Verification items for the finished model (mm, model axes). Face numbers are marked on the shaded views. A direction names the side the tool comes from. Coordinates: 2 decimals unless noted, no trailing zeros. Write each loop counter-clockwise with the first axis right and the second up, starting at its lowest first coordinate (ties: lowest second). Pieces come first, ordered by that corner, then holes. Notation, with made-up numbers: (-22.75, 25) -> (10.25, 25) arc R21 ccw to (10.25, 54) -> close; hole circle Ø7 at (43.5, -18). An arc over 180 degrees is marked (long way). Write item = value, one per line. Start each with the question number.
(1) Gauge pin test, flat ends, axial feed: pin 1 Ø2 at (x, z) = (13.5, 20) entering from -Y; pin 2 Ø5 at (y, z) = (4, 11.5) entering from +X; pin 3 Ø3 at (x, z) = (-13.5, 13.5) entering from +Y; pin 4 Ø12.5 at (x, z) = (-28, 10.5) entering from +Y. Record the tip position at first contact, or that the pin passes through.
(2) Material ranges on probe 1 along Y at (x, z) = (1.8, 9); probe 2 along Y at (x, z) = (-35, 18); probe 3 along Z at (x, y) = (17.5, 1), recorded low to high. Write a range as [from, to].
(3) Mould release check, pull along Z, two halves, no side actions. Record for the marked faces 4, 5, 6 and 7: released by +Z, released by -Z, zero draft, split by the parting line, or undercut.
(4) Section check C-C (x = 7). Record the cut outline in (y, z), plus the area to 3 significant figures.
(5) Section check A-A (x = -23). Record the cut outline in (y, z).
(6) Section check D-D (y = -11.5). Record the cut outline in (x, z).
(7) Section check B-B (z = 12.5). Record the cut outline in (x, y), plus the area to 3 significant figures.
(8) Set-up check for the marked faces 1, 2 and 3: record each of +Z, -Z, +X, -X, +Y, -Y from which the full face is reachable in a straight line by a thin tool's end or side.
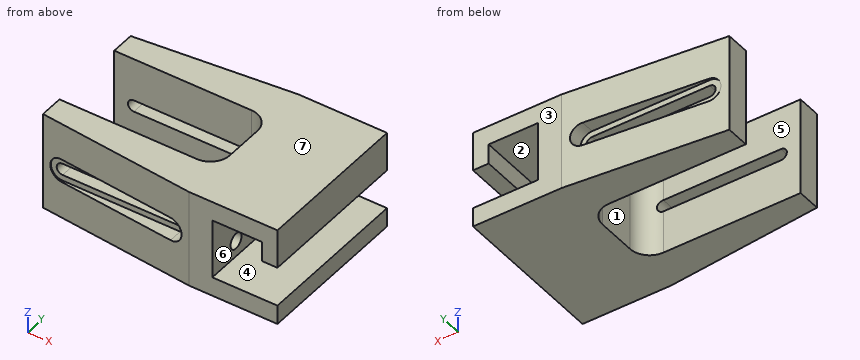
Autodesk Inventor part; units mm, degrees
ref_plane "Work Plane1" through (-40, -10, 25) normal (0, 1, 0) x (1, 0, 0)
ref_plane "YZ Plane" through (0, 0, 0) normal (1, 0, 0) x (0, 1, 0)
ref_plane "XZ Plane" through (0, 0, 0) normal (0, 1, 0) x (-1, 0, 0)
sketch "Sketch1" plane through (0, 0, 0) normal (0, 0, 1) x (1, 0, 0)
  line L0 (-40, 0) -> (0, 0)
  line L1 (0, 0) -> (0, -20)
  line L2 (0, -20) -> (-40, -20)
  line L3 (-40, -20) -> (-40, -26)
  line L4 (-40, -26) -> (0, -30)
  line L5 (0, -30) -> (6, -30)
  line L6 (6, -30) -> (6, 10)
  line L7 (6, 10) -> (0, 10)
  line L8 (0, 10) -> (-40, 6)
  line L9 (-40, 6) -> (-40, 0)
  dimension "d0" = 6
  dimension "d1" = 40
  dimension "d2" = 20
  dimension "d3" = 40
extrude "Extrusion1" add sketch "Sketch1" along normal blind 25
sketch "Sketch2" plane through (6, -30, 0) normal (1, 0, 0) x (0, 0, -1)
  line L0 (0, 40) -> (-25, 40)
  line L1 (0, 0) -> (-25, 0)
  line L2 (-25, 40) -> (-20, 40)
  line L3 (-20, 40) -> (-20, 0)
  line L4 (-20, 0) -> (-25, 0)
  line L5 (-25, 0) -> (-25, 40)
  line L6 (0, 0) -> (-5, 0)
  line L7 (-5, 0) -> (-5, 40)
  line L8 (-5, 40) -> (0, 40)
  line L9 (0, 40) -> (0, 0)
  circle A0 centre (-9, 8.6346) radius 1.7
  line L10 (-2.5, 11.8846) -> (-2.5, 5.3846)
  point P0 (0, 30)
  point P1 (-25, 0)
  point P2 (-5, 0)
  dimension "d6" = 5
  dimension "d7" = 5
  dimension "d30" = 4
  dimension "d31" = 8.6346
extrude "Extrusion2" add sketch "Sketch2" along normal blind 16.6 contours L9 L1 L7 L0 | L3 L1 L5 L0
hole "Hole2" at (6, -21.3654, 9) direction (-1, 0, 0) diameter 4 depth 6
sketch "Sketch3" plane through (0, 0, 0) normal (0, 0, -1) x (-1, 0, 0)
  line L0 (0, 0) -> (0, -20)
  arc A0 (0, -15) -> (5, -20) centre (5, -15) ccw
  arc A1 (5, 0) -> (0, -5) centre (5, -5) ccw
  line L1 (0, -20) -> (40, -20)
  line L2 (40, 0) -> (0, 0)
  dimension "d27" = 5
extrude "Extrusion3" add sketch "Sketch3" against normal up to surface (25 mm away)
sketch "Sketch4" plane through (0, 10, 25) normal (0, 1, 0) x (1, 0, 0)
  line L0 (-5, 12.5) -> (-35, 12.5) construction
  line L1 (-5, 9.5) -> (-35, 9.5)
  line L2 (-35, 15.5) -> (-5, 15.5)
  arc A0 (-5, 9.5) -> (-5, 15.5) centre (-5, 12.5) ccw
  arc A1 (-35, 15.5) -> (-35, 9.5) centre (-35, 12.5) ccw
  line L3 (-40, 25) -> (-40, 0)
  line L4 (0, 25) -> (0, 0)
  point P0 (-20, 12.5)
  point P1 (0, 12.5)
  dimension "d32" = 3
  dimension "d33" = 5
  dimension "d34" = 5
extrude "Extrusion4" cut sketch "Sketch4" against normal blind 4
sketch "Sketch5" plane through (0, 6, 25) normal (0, 1, 0) x (1, 0, 0)
  line L0 (-5, 12.5) -> (-35, 12.5) construction
  line L1 (-5, 14) -> (-35, 14)
  line L2 (-35, 11) -> (-5, 11)
  arc A0 (-5, 11) -> (-5, 14) centre (-5, 12.5) ccw
  arc A1 (-35, 14) -> (-35, 11) centre (-35, 12.5) ccw
  line L3 (-5, 9.5) -> (-35, 9.5)
  arc A2 (-5, 9.5) -> (-5, 15.5) centre (-5, 12.5) ccw
  line L4 (-35, 15.5) -> (-5, 15.5)
  arc A3 (-35, 15.5) -> (-35, 9.5) centre (-35, 12.5) ccw
  point P0 (0, 25)
  point P1 (-20, 12.5)
  dimension "d37" = 1.5
extrude "Extrusion5" cut sketch "Sketch5" against normal blind 10.75 contours A0 L2 A1 L1
ref_plane "Work Plane1" through (-40, -10, 25) normal (0, 1, 0) x (1, 0, 0)
mirror "Mirror1" about plane through (-40, -10, 25) normal (0, 1, 0) of "Extrusion4", "Extrusion5", "Hole2"
sketch "Sketch6" plane through (6, -30, 20) normal (0, 0, -1) x (-1, 0, 0)
  line L0 (0, 40) -> (0, 0)
  line L1 (0, 40) -> (-16.6, 40)
  line L2 (-16.6, 0) -> (-16.6, 40)
  line L3 (0, 0) -> (-16.6, 0)
  line L4 (-16.6, 40) -> (-16.6, 0)
  line L5 (0, 0) -> (-16.6, 0)
  line L6 (-16.6, 40) -> (-12.6, 40)
  line L7 (-12.6, 40) -> (-12.6, 0)
  line L8 (-12.6, 0) -> (-16.6, 0)
  line L9 (-16.6, 0) -> (-16.6, 40)
  point P0 (6, 30)
  dimension "d40" = 4
extrude "Extrusion6" add sketch "Sketch6" along normal blind 5 contours L7 L3 L2 L1
thicken "Thicken1" operation add thickness 0.1 both sides no extend neighbours yes toward (0, 0, 1) faces at (14.4, -3.3333, 20) (11.5333, -3.3333, 5)
properties part number "Z Belt 2"
Response:
q1.pin_1 = -30
q1.pin_2 = 6
q1.pin_3 = 6
q1.pin_4 = 7.82
q2.probe_1 = [-30, -23.37], [-19.37, -0.63], [3.37, 10]
q2.probe_2 = [-26.5, -20], [0, 6.5]
q2.probe_3 = [0, 4.9], [20.1, 25]
q3.face_4 = undercut
q3.face_5 = zero draft
q3.face_6 = undercut
q3.face_7 = released by +Z
q4.outline = (-30, 0) -> (10, 0) -> (10, 4.9) -> (-30, 4.9) -> close; (-30, 20.1) -> (10, 20.1) -> (10, 25) -> (-30, 25) -> close
q4.area = 392 mm2
q5.outline = (-27.7, 0) -> (-20, 0) -> (-20, 11) -> (-26, 11) -> (-26, 9.5) -> (-27.7, 9.5) -> close; (-27.7, 15.5) -> (-26, 15.5) -> (-26, 14) -> (-20, 14) -> (-20, 25) -> (-27.7, 25) -> close; (0, 0) -> (7.7, 0) -> (7.7, 9.5) -> (6, 9.5) -> (6, 11) -> (0, 11) -> close; (0, 14) -> (6, 14) -> (6, 15.5) -> (7.7, 15.5) -> (7.7, 25) -> (0, 25) -> close
q6.outline = (0, 0) -> (22.6, 0) -> (22.6, 4.9) -> (6, 4.9) -> (6, 20.1) -> (18.6, 20.1) -> (18.6, 15) -> (22.6, 15) -> (22.6, 25) -> (0, 25) -> close
q7.outline = (-40, -26) -> (-38, -26.2) -> (-38, -26) -> (-36.5, -26) -> (-36.5, -20) -> (-40, -20) -> close; (-40, 0) -> (-36.5, 0) -> (-36.5, 6) -> (-38, 6) -> (-38, 6.2) -> (-40, 6) -> close; (-3.5, -26) -> (-2, -26) -> (-2, -29.8) -> (0, -30) -> (6, -30) -> (6, 10) -> (0, 10) -> (-2, 9.8) -> (-2, 6) -> (-3.5, 6) -> (-3.5, -0.23) arc R5 cw to (0, -5) -> (0, -15) arc R5 cw to (-3.5, -19.77) -> close
q7.area = 351 mm2
q8.face_1 = +Z, -Z, -X
q8.face_2 = +Y, -Y
q8.face_3 = +Z, -Z, +X, -X, +Y
